CAD build for the part. Positions are in the model's coordinates, mm. A direction names the side the tool comes from. Give positions to 0.01 mm unless a question says otherwise; leave off trailing zeros. Write each loop counter-clockwise with the first axis right and the second up, starting at its lowest first coordinate (ties: lowest second). Pieces come first, ordered by that corner, then holes. Notation, with made-up numbers: (40, 41) - (85, 41) arc R22 ccw to (85, 56) - close; hole circle Ø11 at (57.5, 66). An arc over 180 degrees is marked (long way). Write item = value, one per line. Start each with the question number.
```python
from build123d import *

# Parameters (mm, degrees)
F1_DEPTH = 25.4
F2_SIZE  = 5.08
F3_SIZE  = 5.08


with BuildPart() as f1:
    # F0 (on Front) → F1 (new body)
    with BuildSketch(Plane.XZ):
        Polygon((0, 43.451123), (0, 0), (56.036968, 0), (56.036968, 21.725561), (18.279437, 21.725561), (18.279437, 43.451123), align=None)
    extrude(amount=F1_DEPTH)

    # F2
    f2_edges = [f1.edges().sort_by_distance(p)[0] for p in [
        (56.036968, -12.7, 21.725561),
    ]]
    chamfer(f2_edges, length=F2_SIZE)

    # F3
    f3_edges = [f1.edges().sort_by_distance(p)[0] for p in [
        (18.279437, -12.7, 43.451123),
        (18.279437, -12.7, 21.725561),
        (0, -12.7, 43.451123),
    ]]
    chamfer(f3_edges, length=F3_SIZE)


solid = f1.part
```
1. Cut at B-B (z = 31). Give the cut face in (x, y).
2. Wall check: line 1 along X through (y, z) = (-5, 28.5); line 2 along Z through (x, y) = (48, -5); line 3 along Z through (x, y) = (19.5, -21.5) (3 decimals). Give the ranges that are in metal, low to high.
3. Cut at C-C (x = 49.5). Give the cut face in (y, z), then the cut area to 3 significant figures.
4. Tool access for faces 1 (the flat face through (21, 0, 17)), 2 (the flat face through (37, -13, 21.726)): list every direction of +Z, -Z, +X, -X, +Y, -Y with a clear straight run to the whole face (end or side of a thin tool).
5. Cut at A-A (y = -23.25). Give the cut face in (x, z).
6. Pin check, flat tips, straight feed: pin 1 Ø10 at (x, y) = (31.5, -7) entering from +Z; pin 2 Ø3 at (y, z) = (-7, 22) entering from +X; pin 3 Ø6 at (y, z) = (-9, 34) entering from +X. Stop position of each tip, or through.
Output:
q1.outline = (0, -25.4) - (18.28, -25.4) - (18.28, 0) - (0, 0) - close
q2.line_1 = 0 to 18.28
q2.line_2 = 0 to 21.73
q2.line_3 = 0 to 25.585
q3.outline = (-25.4, 0) - (0, 0) - (0, 21.73) - (-25.4, 21.73) - close
q3.area = 552 mm2
q4.face_1 = +Z, -Z, +X, -X, +Y
q4.face_2 = +Z, +X, +Y, -Y
q5.outline = (0, 0) - (56.04, 0) - (56.04, 16.65) - (50.96, 21.73) - (23.36, 21.73) - (18.28, 26.81) - (18.28, 38.37) - (13.2, 43.45) - (5.08, 43.45) - (0, 38.37) - close
q6.pin_1 = 21.73
q6.pin_2 = 52.18
q6.pin_3 = 18.28
